The model under review builds one solid part; all positions refer to its coordinate system, in mm. A direction names the side the tool comes from. Give positions to 0.01 mm unless a question says otherwise; leave off trailing zeros. Order: outer loops, then holes, each group sorted by start corner. A loop starts at its lowest first (then second) coordinate and runs counter-clockwise, first axis right, second up.
```python
from build123d import *

# Parameters (mm, degrees)
MAINWIRES_R       = 2.5
MAINWIRE_DEPTH    = 10
VCCS_R            = 0.5
VCC_DEPTH         = 6
GROUNDS_R         = 0.5
GROUND_DEPTH      = 6
AS_2_R            = 0.5
EXTRUDE_A_DEPTH   = 6
BS_R              = 0.5
EXTRUDE_B_DEPTH   = 6
ZS_R              = 0.5
EXTRUDE_Z_DEPTH   = 6
A_S_R             = 0.5
EXTRUDE_A_2_DEPTH = 6
B_S_R             = 0.5
EXTRUDE_B_2_DEPTH = 6
Z_S_R             = 0.5
EXTRUDE_Z_2_DEPTH = 6
SHIELDINGS_R      = 2.4
SHIELDINGS_R_2    = 2
SHIELDING_DEPTH   = 4


with BuildPart() as part:
    # MainWireS → MainWire (new body)
    with BuildSketch(Plane(origin=(0, 0, 0), x_dir=(1, 0, 0), z_dir=(0, 1, 0))):
        with Locations(Location((0, 0, 0), (0, 0, 270))):
            Circle(MAINWIRES_R)
    extrude(amount=MAINWIRE_DEPTH)

    # VccS → Vcc (add)
    with BuildSketch(Plane(origin=(0, 10, 0), x_dir=(1, 0, 0), z_dir=(0, 1, 0))):
        with Locations(Location((0, 1.4, 0), (0, 0, 270))):
            Circle(VCCS_R)
    extrude(amount=VCC_DEPTH)

    # GroundS → Ground (add)
    with BuildSketch(Plane(origin=(0, 10, 0), x_dir=(1, 0, 0), z_dir=(0, 1, 0))):
        with Locations(Location((0.989949494, 0.989949494, 0), (0, 0, 270))):
            Circle(GROUNDS_R)
    extrude(amount=GROUND_DEPTH)

    # AS 2 → Extrude A (add)
    with BuildSketch(Plane(origin=(0, 10, 0), x_dir=(1, 0, 0), z_dir=(0, 1, 0))):
        with Locations(Location((1.4, 0, 0), (0, 0, 270))):
            Circle(AS_2_R)
    extrude(amount=EXTRUDE_A_DEPTH)

    # BS → Extrude B (add)
    with BuildSketch(Plane(origin=(0, 10, 0), x_dir=(1, 0, 0), z_dir=(0, 1, 0))):
        with Locations(Location((0.989949494, -0.989949494, 0), (0, 0, 270))):
            Circle(BS_R)
    extrude(amount=EXTRUDE_B_DEPTH)

    # ZS → Extrude Z (add)
    with BuildSketch(Plane(origin=(0, 10, 0), x_dir=(1, 0, 0), z_dir=(0, 1, 0))):
        with Locations(Location((0, -1.4, 0), (0, 0, 270))):
            Circle(ZS_R)
    extrude(amount=EXTRUDE_Z_DEPTH)

    # A-S → Extrude A 2 (add)
    with BuildSketch(Plane(origin=(0, 10, 0), x_dir=(1, 0, 0), z_dir=(0, 1, 0))):
        with Locations(Location((-0.989949494, -0.989949494, 0), (0, 0, 270))):
            Circle(A_S_R)
    extrude(amount=EXTRUDE_A_2_DEPTH)

    # B-S → Extrude B 2 (add)
    with BuildSketch(Plane(origin=(0, 10, 0), x_dir=(1, 0, 0), z_dir=(0, 1, 0))):
        with Locations(Location((-1.4, 0, 0), (0, 0, 270))):
            Circle(B_S_R)
    extrude(amount=EXTRUDE_B_2_DEPTH)

    # Z-S → Extrude Z 2 (add)
    with BuildSketch(Plane(origin=(0, 10, 0), x_dir=(1, 0, 0), z_dir=(0, 1, 0))):
        with Locations(Location((-0.989949494, 0.989949494, 0), (0, 0, 270))):
            Circle(Z_S_R)
    extrude(amount=EXTRUDE_Z_2_DEPTH)

    # ShieldingS → Shielding (add)
    with BuildSketch(Plane(origin=(0, 10, 0), x_dir=(1, 0, 0), z_dir=(0, 1, 0))):
        with Locations(Location((0, 0, 0), (0, 0, 270))):
            Circle(SHIELDINGS_R)
        with Locations(Location((0, 0, 0), (0, 0, 270))):
            Circle(SHIELDINGS_R_2, mode=Mode.SUBTRACT)
    extrude(amount=SHIELDING_DEPTH)


solid = part.part
```
1. Take a section at A-A (y = 14.75). Write out the cut boundary in (x, z).
2. Take a section at C-C (y = 11.25). Count the separate pieces of the cut face and the enclosed holes in it, and give its area (3 significant figures).
3. Insertion check: pin 1 (1.5 mm diameter, centred on x = 1.5, y = 14.5, fed in from -Z). The pin has a flat end and moves straight along its axis. Give the tip position at first contact, or say it passes through.
4. To check wall thickness, follow line 1 (Z direction, x = 0.3, y = 11.25); line 2 (Y direction, x = -0.85, z = 0.1); line 3 (Y direction, x = -1.5, z = -1.7). State the ranges of each line that lie inside material, in increasing order.
5. Take a section at D-D (x = 0). Write out the cut boundary in (y, z).
6. Take a section at B-B (z = 0). Write out the cut boundary in (x, y).
7. Draft analysis for pull direction Z (two halves, no side actions). For faces 3 (the flat face through (1, 16, 1)), 4 (the cylindrical face through (-0.444, 12.958, 1.631)), 5 (the cylindrical face through (-2.44, 4.93, -0.54)), 6 (the cylindrical face through (-0.3, 13, -1.8)), state which applies: pulls with the +Z half, pulls with the -Z half, needs draft (parallel to the pull), parting line crosses it, or undercut.
8. For faces 1 (the cylindrical face through (-0.904, 12.958, -0.065)), 2 (the flat face through (1.4, 16, 0)), list the 3-axis set-ups (+Z, -Z, +X, -X, +Y, -Y) from which the entire face can be reached by the end or side of a thin tool; tool diameter is ignored.
Answer:
1. outline: circle Ø1 at (-1.4, 0); circle Ø1 at (-0.99, -0.99); circle Ø1 at (-0.99, 0.99); circle Ø1 at (0, -1.4); circle Ø1 at (0, 1.4); circle Ø1 at (0.99, -0.99); circle Ø1 at (0.99, 0.99); circle Ø1 at (1.4, 0)
2. separate pieces: 9
2. enclosed holes: 1
2. area: 11.8 mm2
3. pin 1: stops at z = -2.21
4. line 1: z = -2.38 to -1.98, -1.8 to -1, 1 to 1.8, 1.98 to 2.38
4. line 2: y = 0 to 10
4. line 3: y = 0 to 14
5. outline: (0, -2.5) - (10, -2.5) - (10, -2.4) - (14, -2.4) - (14, -2) - (10, -2) - (10, -1.9) - (16, -1.9) - (16, -0.9) - (10, -0.9) - (10, 0.9) - (16, 0.9) - (16, 1.9) - (10, 1.9) - (10, 2) - (14, 2) - (14, 2.4) - (10, 2.4) - (10, 2.5) - (0, 2.5) - close
6. outline: (-2.5, 0) - (2.5, 0) - (2.5, 10) - (2.4, 10) - (2.4, 14) - (2, 14) - (2, 10) - (1.9, 10) - (1.9, 16) - (0.9, 16) - (0.9, 10) - (-0.9, 10) - (-0.9, 16) - (-1.9, 16) - (-1.9, 10) - (-2, 10) - (-2, 14) - (-2.4, 14) - (-2.4, 10) - (-2.5, 10) - close
7. face 3: needs draft
7. face 4: undercut
7. face 5: parting line crosses it
7. face 6: undercut
8. face 1: +Y
8. face 2: +Z, -Z, +X, -X, +Y
